from build123d import *

# Parameters (mm, degrees)
SCHIZZO1_R                   = 11
ESTRUSIONE_ESTRUSIONE1_DEPTH = 9
ESTRUSIONE_ESTRUSIONE2_DEPTH = 8
RACCORDO1_R                  = 1
SCHIZZO5_R                   = 8
SCHIZZO4_R                   = 5


with BuildPart() as part:
    # Schizzo1 → Estrusione-Estrusione1 (new body)
    with BuildSketch(Plane.XY):
        Circle(SCHIZZO1_R)
    extrude(amount=ESTRUSIONE_ESTRUSIONE1_DEPTH)

    # Schizzo2 → Estrusione-Estrusione2 (add)
    with BuildSketch(Plane(origin=(0, 0, 0), x_dir=(-1, 0, 0), z_dir=(0, 0, -1))):
        Polygon((-19.551988484, -1.747306402), (-8.26278251, -17.806171922), (11.289205974, -16.058865521), (19.551988484, 1.747306402), (8.26278251, 17.806171922), (-11.289205974, 16.058865521), align=None)
    extrude(amount=ESTRUSIONE_ESTRUSIONE2_DEPTH)

    # Raccordo1
    raccordo1_edges = [part.edges().sort_by_distance(p)[0] for p in [
        (1.513211732, 16.932518721, -8),
        (15.420597229, 7.155779559, -8),
        (13.907385497, -9.776739162, -8),
        (-1.513211732, -16.932518721, -8),
        (-15.420597229, -7.155779559, -8),
        (-13.907385497, 9.776739162, -8),
    ]]
    fillet(raccordo1_edges, radius=RACCORDO1_R)

    # Schizzo5 → Loft1 section 0
    with BuildSketch(Plane.XY.offset(9)):
        Circle(SCHIZZO5_R)
    # Schizzo4 → Loft1 section 1
    with BuildSketch(Plane.XY.offset(12)):
        Circle(SCHIZZO4_R)
    loft()


solid = part.part
Read the model definition and answer for the solid it produces. Units are mm, in the model's axes. A direction names the side the tool comes from. Round coordinates to 2 decimals unless told otherwise and drop trailing zeros. Order: outer loops, then holes, each group sorted by start corner. A loop starts at its lowest first (then second) coordinate and runs counter-clockwise, first axis right, second up. Notation, with made-up numbers: (-35.75, 54) - (10.25, 54) arc R18 cw to (10.25, 79) - close; hole circle Ø6 at (-14.5, 24). An arc over 180 degrees is marked (long way). Use one line per item in the form item = value. Start each with the question number.
(1) For faces 1 (the face through (-15.206, -6.905, -7.715)), 2 (the face through (-8, -8, 0)), determine the directions among +Z, -Z, +X, -X, +Y, -Y from which every point of the face is accessible in a straight line to the end or side of a thin tool.
(2) The part is cut by section A-A (z = -5.5). Give the vertices of the cut face in (x, y).
(3) The part is cut by section B-B (z = 6). Give the vertices of the cut face in (x, y).
(4) Flat-ended cylindrical pins translate along their axes: pin 1 Ø10 at (x, z) = (6.5, 8.5) entering from +Y; pin 2 Ø1.5 at (x, y) = (10.5, -7) entering from +Z; pin 3 Ø4 at (x, y) = (-1, -10) entering from +Z. Find the tip coordinate at first contact, or state that the pin passes through.
(5) Find the intervals of material crossed by line 1 along Z through (x, y) = (8, 14.5); line 2 along Z through (x, y) = (-1.5, -10); line 3 along X through (y, z) = (12, -6), in increasing order. Write a range as from..to.
Checked values:
q1.face_1 = -Z, -X, -Y
q1.face_2 = +Z
q2.outline = (-19.55, 1.75) - (-11.29, -16.06) - (8.26, -17.81) - (19.55, -1.75) - (11.29, 16.06) - (-8.26, 17.81) - close
q3.outline = circle Ø22 at (0, 0)
q4.pin_1 = 10.9
q4.pin_2 = 0
q4.pin_3 = 9
q5.line_1 = -8..0
q5.line_2 = -8..9
q5.line_3 = -12.34..13.17
